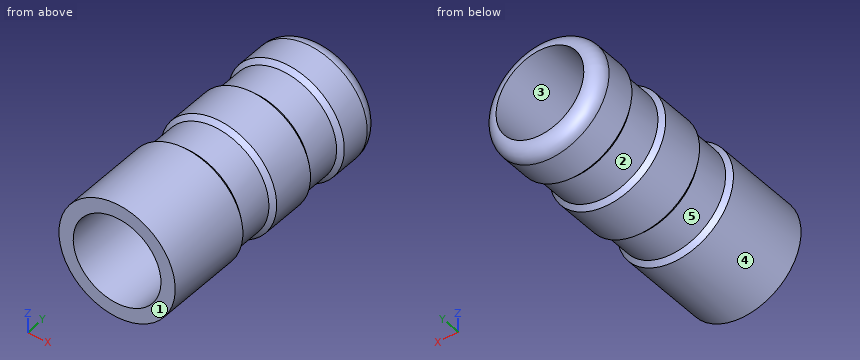
from build123d import *

# Parameters (mm, degrees)
SKETCH1_R           = 16.8275
SKETCH1_R_2         = 12.7
BOSS_EXTRUDE1_DEPTH = 76.2
FILLET1_R           = 4.1275


with BuildPart() as part:
    # Sketch1 → Boss-Extrude1 (new body)
    with BuildSketch(Plane(origin=(0, 0, 0), x_dir=(1, 0, 0), z_dir=(0, 1, 0))):
        with Locations(Location((0, 0, 0), (0, 0, 90))):
            Circle(SKETCH1_R)
        with Locations(Location((0, 0, 0), (0, 0, 90))):
            Circle(SKETCH1_R_2, mode=Mode.SUBTRACT)
    extrude(amount=BOSS_EXTRUDE1_DEPTH)

    # Fillet1
    fillet1_edges = [part.edges().sort_by_distance(p)[0] for p in [
        (0, 76.2, 16.8275),
    ]]
    fillet(fillet1_edges, radius=FILLET1_R - 0.0001)  # a hair under: the kernel refuses the full size

    # Sketch2 → Cut-Revolve1 (revolve, cut)
    with BuildSketch(Plane.XY, mode=Mode.PRIVATE) as cut_revolve1_sk:
        Polygon((16.8275, 63.5), (15.5575, 62.23), (15.5575, 52.07), (16.8275, 50.8), align=None)
        Polygon((16.8275, 38.1), (15.5575, 36.83), (15.5575, 26.67), (16.8275, 25.4), align=None)
    revolve(cut_revolve1_sk.sketch.rotate(Axis((0, 0, 0), (0, 1, 0)), 90), axis=Axis((0, 0, 0), (0, 1, 0)), mode=Mode.SUBTRACT)


solid = part.part
For this review, take the finished solid that the model builds, in its own axes (mm). Face numbers are marked on the shaded views. A direction names the side the tool comes from. Round coordinates to 2 decimals unless told otherwise and drop trailing zeros. Loops run counter-clockwise (first coordinate to the right, second up) from the corner with the lowest first, then second, coordinate; pieces in that order, holes last. Notation, with made-up numbers: (9, -25) - (39, -25) arc R18 cw to (39, -12) - close; hole circle Ø10 at (53, 51.25). An arc over 180 degrees is marked (long way). Answer as CSV lines item,"result".
(1) Insertion check: P1, Ø2, axis at y = 52, z = -9.5, coming from the +X side; P2, Ø4, axis at x = 9.5, y = 42.5, coming from the -Z side; P3, Ø6, axis at x = -7, y = 10.5, coming from the +Z side. Each pin has a flat end and moves straight along its axis. Give the tip position at first contact, or say it passes through.
Checked values:
P1,"stops at x = 13.82"
P2,"stops at z = -15.06"
P3,"stops at z = 16.35"
(2) Consider section D-D on y = 16.5. Give the boundary of the cut face in (x, z) (1 decimal), then the cut area to 3 significant figures.
Checked values:
outline,"circle Ø33.7 at (0, 0); hole circle Ø25.4 at (0, 0)"
area,"383 mm2"
(3) Mouldability with a two-part tool opening along Z and no side actions: class the marked faces 1, 2 and 3 as +Z half, -Z half, draft (parallel to the pull), parting line (faces both ways), or undercut.
Checked values:
face 1,"draft"
face 2,"parting line"
face 3,"undercut"
(4) Tool access review of the marked faces 4 and 5: name each direction out of +Z, -Z, +X, -X, +Y, -Y from which nothing blocks a thin tool from reaching the whole face with its end or side.
Checked values:
face 4,"+Y, -Y"
face 5,"none"
(5) Wall thickness on line 1 (X direction, y = 46, z = 0); line 2 (X direction, y = 28.5, z = 0); line 3 (Y direction, x = -13, z = -9): over which ranges is each line inside the solid? List them lowest first.
Checked values:
line 1,"x = -16.83 to -12.7, 12.7 to 16.83"
line 2,"x = -15.56 to -12.7, 12.7 to 15.56"
line 3,"y = 0 to 26.42, 37.08 to 51.82, 62.48 to 74.78"
(6) Consider section C-C on y = 58. Give the boundary of the cut face in (x, z) (1 decimal), then the cut area to 3 significant figures.
Checked values:
outline,"circle Ø31.1 at (0, 0); hole circle Ø25.4 at (0, 0)"
area,"254 mm2"
